Build history of the part. All positions in model axes, mm. Give positions to 0.01 mm unless a question says otherwise; leave off trailing zeros. Loops run counter-clockwise (first coordinate to the right, second up) from the corner with the lowest first, then second, coordinate; pieces in that order, holes last. Notation, with made-up numbers: M -16.75,2 L 11.25,2 A9 ccw 11.25,16 Z; hole C 52,-9 d11. An arc over 180 degrees is marked long. Answer in a Markdown table with one row per item. Add a question column.
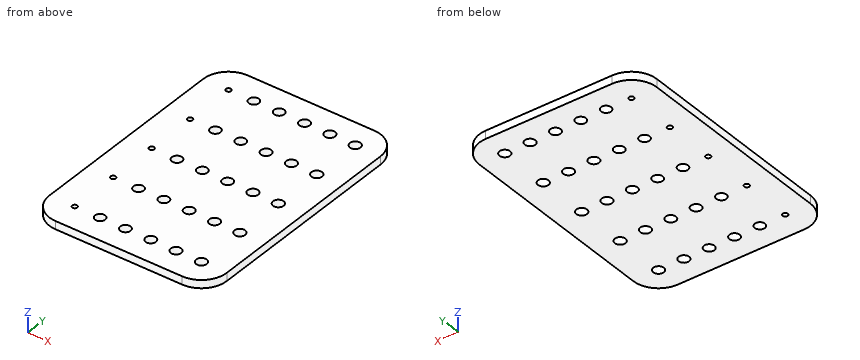
```python
from build123d import *

# Parameters (mm, degrees)
SKETCH1_W           = 70
SKETCH1_H           = 20
SKETCH1_R           = 2
SKETCH1_R_2         = 2.025
SKETCH1_R_3         = 2.05
SKETCH1_R_4         = 2.1
SKETCH1_R_5         = 2.075
SKETCH1_R_6         = 1
BOSS_EXTRUDE1_DEPTH = 3.175
LPATTERN1_COUNT     = 5
LPATTERN1_PITCH     = 20
FILLET1_R           = 10


with BuildPart() as part:
    # Sketch1 → Boss-Extrude1 (new body)
    with BuildSketch(Plane.XY):
        with Locations((15, 0)):
            Rectangle(SKETCH1_W, SKETCH1_H)
        Circle(SKETCH1_R, mode=Mode.SUBTRACT)
        with Locations((10, 0)):
            Circle(SKETCH1_R_2, mode=Mode.SUBTRACT)
        with Locations((20, 0)):
            Circle(SKETCH1_R_3, mode=Mode.SUBTRACT)
        with Locations((40, 0)):
            Circle(SKETCH1_R_4, mode=Mode.SUBTRACT)
        with Locations((30, 0)):
            Circle(SKETCH1_R_5, mode=Mode.SUBTRACT)
        with Locations((-10, 0)):
            Circle(SKETCH1_R_6, mode=Mode.SUBTRACT)
    boss_extrude1 = extrude(amount=BOSS_EXTRUDE1_DEPTH)

    # LPattern1: Boss-Extrude1 ×5
    with Locations(*[(0, -i * LPATTERN1_PITCH, 0) for i in range(1, LPATTERN1_COUNT)]):
        add(boss_extrude1)

    # Fillet1
    fillet1_edges = [part.edges().sort_by_distance(p)[0] for p in [
        (50, -90, 1.5875),
        (-20, -90, 1.5875),
        (-20, 10, 1.5875),
        (50, 10, 1.5875),
    ]]
    fillet(fillet1_edges, radius=FILLET1_R)


solid = part.part
```
(1) Slice it at B-B, the plane x = 20. Give the cut face in (y, z) (3 decimals), then the cut area to 3 significant figures.
(2) Wall check: line 1 (Y direction, x = -10, z = 1.95); line 2 (Y direction, x = 20, z = 2.5); line 3 (X direction, y = -81.5, z = 2.8). Give the ranges that are in metal, low to high.
(3) Slice it at A-A, the plane y = -20. Give the cut face in (x, z) (3 decimals).
(4) Pin check, flat tip, straight feed: pin 1 (3.5 mm diameter, centred on x = 20, y = -20, fed in from -Z). Stop position of the tip, or through.
(5) Slice it at C-C, the plane z = 1.95. State how many separate pieces and enclosed holes the cut face has, then the cut area to 3 significant figures.
(6) Slice it at D-D, the plane x = -15. Give the cut face in (y, z) (3 decimals).
Solution:
| question | item | result |
|---|---|---|
| 1 | outline | M -90,0 L -82.05,0 L -82.05,3.175 L -90,3.175 Z; M -77.95,0 L -62.05,0 L -62.05,3.175 L -77.95,3.175 Z; M -57.95,0 L -42.05,0 L -42.05,3.175 L -57.95,3.175 Z; M -37.95,0 L -22.05,0 L -22.05,3.175 L -37.95,3.175 Z; M -17.95,0 L -2.05,0 L -2.05,3.175 L -17.95,3.175 Z; M 2.05,0 L 10,0 L 10,3.175 L 2.05,3.175 Z |
| 1 | area | 252 mm^2 |
| 2 | line 1 | -90 to -81, -79 to -61, -59 to -41, -39 to -21, -19 to -1, 1 to 10 |
| 2 | line 2 | -90 to -82.05, -77.95 to -62.05, -57.95 to -42.05, -37.95 to -22.05, -17.95 to -2.05, 2.05 to 10 |
| 2 | line 3 | -19.89 to -1.32, 1.32 to 8.64, 11.36 to 18.6, 21.4 to 28.57, 31.43 to 38.53, 41.47 to 49.89 |
| 3 | outline | M -20,0 L -11,0 L -11,3.175 L -20,3.175 Z; M -9,0 L -2,0 L -2,3.175 L -9,3.175 Z; M 2,0 L 7.975,0 L 7.975,3.175 L 2,3.175 Z; M 12.025,0 L 17.95,0 L 17.95,3.175 L 12.025,3.175 Z; M 22.05,0 L 27.925,0 L 27.925,3.175 L 22.05,3.175 Z; M 32.075,0 L 37.9,0 L 37.9,3.175 L 32.075,3.175 Z; M 42.1,0 L 50,0 L 50,3.175 L 42.1,3.175 Z |
| 4 | pin 1 | through |
| 5 | separate pieces | 1 |
| 5 | enclosed holes | 30 |
| 5 | area | 6,570 mm^2 |
| 6 | outline | M -88.66,0 L 8.66,0 L 8.66,3.175 L -88.66,3.175 Z |
